```python
from build123d import *

# Parameters (mm, degrees)
F0_W     = 24
F0_H     = 60
F1_DEPTH = 10
F2_W     = 8
F2_H     = 4
F3_DEPTH = 25
F4_W     = 5
F4_H     = 5
F5_DEPTH = 60
F6_W     = 5
F6_H     = 5
F7_DEPTH = 60


with BuildPart() as f1:
    # F0 (on Top) → F1 (new body)
    with BuildSketch(Plane.XY):
        Rectangle(F0_W, F0_H)
    extrude(amount=F1_DEPTH)

    # F2 (on face) → F3 (cut)
    with BuildSketch(Plane.XY.offset(10)):
        with Locations((0, 23)):
            Rectangle(F2_W, F2_H)
    extrude(amount=-F3_DEPTH, mode=Mode.SUBTRACT)

    # F4 (on face) → F5 (join)
    with BuildSketch(Plane.YZ.offset(12)):
        with Locations((-22.5, 5)):
            Rectangle(F4_W, F4_H)
    extrude(amount=F5_DEPTH)

    # F6 (on face) → F7 (join)
    with BuildSketch(Plane(origin=(-12, 0, 0), x_dir=(0, -1, 0), z_dir=(-1, 0, 0))):
        with Locations((22.5, 5)):
            Rectangle(F6_W, F6_H)
    extrude(amount=F7_DEPTH)


solid = f1.part
```
Verification items for the finished model (mm, model axes). A direction names the side the tool comes from. Coordinates: 2 decimals unless noted, no trailing zeros. Write each loop counter-clockwise with the first axis right and the second up, starting at its lowest first coordinate (ties: lowest second). Pieces come first, ordered by that corner, then holes. Notation, with made-up numbers: M 86.5,15 L 114.5,15 A17 ccw 114.5,33 Z; hole C -7,69.5 d4. An arc over 180 degrees is marked long. One line per item, written item: value.
Item 1: Section check B-B, the plane z = 5. Record the boundary of the cut face in (x, y).
Check sheet entries:
outline: M -72,-25 L -12,-25 L -12,-30 L 12,-30 L 12,-25 L 72,-25 L 72,-20 L 12,-20 L 12,30 L -12,30 L -12,-20 L -72,-20 Z; hole M -4,21 L 4,21 L 4,25 L -4,25 Z
Item 2: Section check C-C, the plane y = -23. Record the boundary of the cut face in (x, z), plus the area to 3 significant figures.
Check sheet entries:
outline: M -72,2.5 L -12,2.5 L -12,0 L 12,0 L 12,2.5 L 72,2.5 L 72,7.5 L 12,7.5 L 12,10 L -12,10 L -12,7.5 L -72,7.5 Z
area: 840 mm^2
Item 3: Section check A-A, the plane y = 23. Record the boundary of the cut face in (x, z), plus the area to 3 significant figures.
Check sheet entries:
outline: M -12,0 L -4,0 L -4,10 L -12,10 Z; M 4,0 L 12,0 L 12,10 L 4,10 Z
area: 160 mm^2
Item 4: Section check D-D, the plane x = -51.5. Record the boundary of the cut face in (y, z).
Check sheet entries:
outline: M -25,2.5 L -20,2.5 L -20,7.5 L -25,7.5 Z
Item 5: Scan lines: line 1 along X through (y, z) = (26, 5); line 2 along Y through (x, z) = (54.5, 5); line 3 along Z through (x, y) = (27.5, -21). Record each from-to range of solid material in increasing order.
Check sheet entries:
line 1: x = -12 to 12
line 2: y = -25 to -20
line 3: z = 2.5 to 7.5
Item 6: Gauge pin test, flat ends, axial feed: pin 1 Ø5.5 at (x, z) = (38, 4) entering from -Y; pin 2 Ø1.5 at (x, y) = (52, -22.5) entering from +Z; pin 3 Ø5.5 at (x, z) = (32, 4) entering from +Y. Record the tip position at first contact, or that the pin passes through.
Check sheet entries:
pin 1: stops at y = -25
pin 2: stops at z = 7.5
pin 3: stops at y = -20
Item 7: Mould release check, pull along Y, two halves, no side actions. Record for faces 6 (the flat face through (4, 23, 5)), 7 (the flat face through (-4, 23, 5)), 8 (the flat face through (42, -20, 5)), 9 (the flat face through (72, -23, 5)): pulls with the +Y half, pulls with the -Y half, needs draft (parallel to the pull), parting line crosses it, or undercut.
Check sheet entries:
face 6: undercut
face 7: undercut
face 8: pulls with the +Y half
face 9: needs draft
Item 8: Access from +Z, -Z, +X, -X, +Y, -Y to the whole of each face (thin tool, end or side, straight path). Record for faces 1 (the flat face through (-42, -22, 2.5)), 2 (the flat face through (0, 25, 5)), 3 (the flat face through (42, -23, 2.5)), 4 (the flat face through (-42, -22, 7.5)), 5 (the flat face through (-42, -20, 5)).
Check sheet entries:
face 1: -Z, -X, +Y, -Y
face 2: +Z, -Z
face 3: -Z, +X, +Y, -Y
face 4: +Z, -X, +Y, -Y
face 5: +Z, -Z, -X, +Y
